Can you work these out from the model? Positions are in its coordinate system, mm. A direction names the side the tool comes from. Round coordinates to 2 decimals unless told otherwise and drop trailing zeros. Order: outer loops, then holes, each group sorted by start corner. A loop starts at its lowest first (then second) coordinate and runs counter-clockwise, first axis right, second up. Notation, with made-up numbers: (-37.5, -25.5) -> (-20.5, -25.5) arc R24 cw to (-20.5, -4.5) -> close; hole circle Ø9 at (64, 29.25). An arc over 180 degrees is marked (long way). One line per item, written item: value.
```python
from build123d import *

# Parameters (mm, degrees)
ESTRUSIONE_ESTRUSIONE1_DEPTH = 7.5
ESTRUSIONE_ESTRUSIONE2_DEPTH = 4
TAGLIO_ESTRUSIONE1_DEPTH     = 198.380910943
TAGLIO_ESTRUSIONE2_DEPTH     = 198.380910943
RACCORDO1_R                  = 25
TAGLIO_ESTRUSIONE3_DEPTH     = 7.5
TAGLIO_ESTRUSIONE4_DEPTH     = 7.5
SCHIZZO6_R                   = 3
TAGLIO_ESTRUSIONE5_DEPTH     = 198.380910943


with BuildPart() as part:
    # Schizzo1 → Estrusione-Estrusione1 (new, symmetric)
    with BuildSketch(Plane.XY):
        with BuildLine():
            Line((14.5, 182.011383906), (14.5, -37.988616094))
            ThreePointArc((14.5, -37.988616094), (0, -52.488616094), (-14.5, -37.988616094))
            Line((-14.5, -37.988616094), (-14.5, 182.011383906))
            ThreePointArc((-14.5, 182.011383906), (0, 196.511383906), (14.5, 182.011383906))
        make_face()
    extrude(amount=ESTRUSIONE_ESTRUSIONE1_DEPTH, both=True)

    # Schizzo2 → Estrusione-Estrusione2 (add, symmetric)
    with BuildSketch(Plane.XY):
        with BuildLine():
            Line((13, -40.066616094), (13, -56.066616094))
            ThreePointArc((13, -56.066616094), (0, -69.066616094), (-13, -56.066616094))
            Line((-13, -56.066616094), (-13, -40.066616094))
            ThreePointArc((-13, -40.066616094), (0, -27.066616094), (13, -40.066616094))
        make_face()
    extrude(amount=ESTRUSIONE_ESTRUSIONE2_DEPTH, both=True)

    # Schizzo4 → Taglio-Estrusione1 (cut, through all)
    with BuildSketch(Plane.XY.offset(4)):
        with BuildLine():
            Line((5.29445937, -51.487456784), (14.5, -37.988616094))
            Line((14.5, -37.988616094), (21.494330869, -44.738036439))
            Line((21.494330869, -44.738036439), (5.386515672, -60.537124892))
            ThreePointArc((5.386515672, -60.537124892), (0.071202698, -63.066253954), (-5.29445937, -60.645775404))
            Line((-5.29445937, -60.645775404), (-28.596127717, -39.453615031))
            Line((-28.596127717, -39.453615031), (-14.5, -31.562211214))
            Line((-14.5, -31.562211214), (-3.845832517, -50.217721134))
            ThreePointArc((-3.845832517, -50.217721134), (0.963165144, -49.133196093), (5.29445937, -51.487456784))
        make_face()
    taglio_estrusione1 = extrude(amount=TAGLIO_ESTRUSIONE1_DEPTH, mode=Mode.SUBTRACT)

    # Specchia1: Taglio-Estrusione1 across plane
    add(taglio_estrusione1.mirror(Plane.XY), mode=Mode.SUBTRACT)

    # Schizzo5 → Taglio-Estrusione2 (cut, through all)
    with BuildSketch(Plane.XY.offset(4)):
        Polygon((-13, -44.411232383), (-13, -34.188720036), (-15.056335757, -30.588064032), (-15.056335757, -43.619366988), align=None)
        Polygon((13, -44.411232383), (13, -40.188189356), (17.407959402, -33.724436261), (17.407959402, -44.411232383), align=None)
    extrude(amount=-TAGLIO_ESTRUSIONE2_DEPTH, mode=Mode.SUBTRACT)

    # Raccordo1
    # the kernel refuses this fillet: 25 mm, written as the material it takes off along each edge
    with BuildSketch(Plane(origin=(-14.5, -31.562211214, -24.089497944), x_dir=(0.4959240379913526, -0.8683659070589721, 0), z_dir=(0, 0, 1))) as raccordo1_piece_1_section:
        with BuildLine():
            CenterArc((RACCORDO1_R * 0.26543196711, RACCORDO1_R), RACCORDO1_R, 240.269299078, 29.730700922)
            Line((-RACCORDO1_R * 0.230492070882, RACCORDO1_R * 0.131634092941), (0, 0))
            Line((0, 0), (RACCORDO1_R * 0.26543196711, 0))
        make_face()
    raccordo1_piece_1 = extrude(amount=48.178995889, mode=Mode.PRIVATE)
    raccordo1_piece_1 = split(raccordo1_piece_1, bisect_by=Plane(origin=(-13, -35.788331904, -14.044748972), z_dir=(1, 0, 0)), keep=Keep.TOP, mode=Mode.PRIVATE)
    raccordo1_piece_1 = split(raccordo1_piece_1, bisect_by=Plane(origin=(-12.28179921, -35.788331904, -4), z_dir=(0, 0, -1)), keep=Keep.TOP, mode=Mode.PRIVATE)
    add(raccordo1_piece_1, mode=Mode.SUBTRACT)
    with BuildSketch(Plane(origin=(-14.5, -31.562211214, -24.089497944), x_dir=(0.4959240379913526, -0.8683659070589721, 0), z_dir=(0, 0, 1))) as raccordo1_piece_2_section:
        with BuildLine():
            CenterArc((RACCORDO1_R * 0.26543196711, RACCORDO1_R), RACCORDO1_R, 240.269299078, 29.730700922)
            Line((-RACCORDO1_R * 0.230492070882, RACCORDO1_R * 0.131634092941), (0, 0))
            Line((0, 0), (RACCORDO1_R * 0.26543196711, 0))
        make_face()
    raccordo1_piece_2 = extrude(amount=48.178995889, mode=Mode.PRIVATE)
    raccordo1_piece_2 = split(raccordo1_piece_2, bisect_by=Plane(origin=(-13, -30.370530988, -14.044748972), z_dir=(-1, 0, 0)), keep=Keep.TOP, mode=Mode.PRIVATE)
    raccordo1_piece_2 = split(raccordo1_piece_2, bisect_by=Plane(origin=(-14.266276842, -30.370530988, -4), z_dir=(0, 0, -1)), keep=Keep.TOP, mode=Mode.PRIVATE)
    add(raccordo1_piece_2, mode=Mode.SUBTRACT)
    with BuildSketch(Plane(origin=(-14.5, -31.562211214, -24.089497944), x_dir=(0.4959240379913526, -0.8683659070589721, 0), z_dir=(0, 0, 1))) as raccordo1_piece_3_section:
        with BuildLine():
            CenterArc((RACCORDO1_R * 0.26543196711, RACCORDO1_R), RACCORDO1_R, 240.269299078, 29.730700922)
            Line((-RACCORDO1_R * 0.230492070882, RACCORDO1_R * 0.131634092941), (0, 0))
            Line((0, 0), (RACCORDO1_R * 0.26543196711, 0))
        make_face()
    raccordo1_piece_3 = extrude(amount=48.178995889, mode=Mode.PRIVATE)
    raccordo1_piece_3 = split(raccordo1_piece_3, bisect_by=Plane(origin=(-14.266276842, -30.370530988, 4), z_dir=(0, 0, -1)), keep=Keep.TOP, mode=Mode.PRIVATE)
    raccordo1_piece_3 = split(raccordo1_piece_3, bisect_by=Plane(origin=(-13, -30.370530988, 0), z_dir=(-1, 0, 0)), keep=Keep.TOP, mode=Mode.PRIVATE)
    raccordo1_piece_3 = split(raccordo1_piece_3, bisect_by=Plane(origin=(-14.266276842, -30.370530988, -4), z_dir=(0, 0, 1)), keep=Keep.TOP, mode=Mode.PRIVATE)
    add(raccordo1_piece_3, mode=Mode.SUBTRACT)
    with BuildSketch(Plane(origin=(-14.5, -31.562211214, -24.089497944), x_dir=(0.4959240379913526, -0.8683659070589721, 0), z_dir=(0, 0, 1))) as raccordo1_piece_4_section:
        with BuildLine():
            CenterArc((RACCORDO1_R * 0.26543196711, RACCORDO1_R), RACCORDO1_R, 240.269299078, 29.730700922)
            Line((-RACCORDO1_R * 0.230492070882, RACCORDO1_R * 0.131634092941), (0, 0))
            Line((0, 0), (RACCORDO1_R * 0.26543196711, 0))
        make_face()
    raccordo1_piece_4 = extrude(amount=48.178995889, mode=Mode.PRIVATE)
    raccordo1_piece_4 = split(raccordo1_piece_4, bisect_by=Plane(origin=(-12.28179921, -35.788331904, 4), z_dir=(0, 0, 1)), keep=Keep.TOP, mode=Mode.PRIVATE)
    raccordo1_piece_4 = split(raccordo1_piece_4, bisect_by=Plane(origin=(-13, -35.788331904, 14.044748972), z_dir=(1, 0, 0)), keep=Keep.TOP, mode=Mode.PRIVATE)
    add(raccordo1_piece_4, mode=Mode.SUBTRACT)
    with BuildSketch(Plane(origin=(-14.5, -31.562211214, -24.089497944), x_dir=(0.4959240379913526, -0.8683659070589721, 0), z_dir=(0, 0, 1))) as raccordo1_piece_5_section:
        with BuildLine():
            CenterArc((RACCORDO1_R * 0.26543196711, RACCORDO1_R), RACCORDO1_R, 240.269299078, 29.730700922)
            Line((-RACCORDO1_R * 0.230492070882, RACCORDO1_R * 0.131634092941), (0, 0))
            Line((0, 0), (RACCORDO1_R * 0.26543196711, 0))
        make_face()
    raccordo1_piece_5 = extrude(amount=48.178995889, mode=Mode.PRIVATE)
    raccordo1_piece_5 = split(raccordo1_piece_5, bisect_by=Plane(origin=(-14.266276842, -30.370530988, 4), z_dir=(0, 0, 1)), keep=Keep.TOP, mode=Mode.PRIVATE)
    raccordo1_piece_5 = split(raccordo1_piece_5, bisect_by=Plane(origin=(-13, -30.370530988, 14.044748972), z_dir=(-1, 0, 0)), keep=Keep.TOP, mode=Mode.PRIVATE)
    add(raccordo1_piece_5, mode=Mode.SUBTRACT)
    with BuildSketch(Plane(origin=(14.5, -37.988616094, 26.782481556), x_dir=(0, 1, 0), z_dir=(0, 0, -1))) as raccordo1_piece_6_section:
        with BuildLine():
            CenterArc((RACCORDO1_R * 0.308519704891, -RACCORDO1_R), RACCORDO1_R, 90, 34.292050498)
            Line((-RACCORDO1_R * 0.254891721625, -RACCORDO1_R * 0.173823527041), (0, 0))
            Line((0, 0), (RACCORDO1_R * 0.308519704891, 0))
        make_face()
    raccordo1_piece_6 = extrude(amount=53.564963111, mode=Mode.PRIVATE)
    raccordo1_piece_6 = split(raccordo1_piece_6, bisect_by=Plane(origin=(14.242102238, -36.251699178, 4), z_dir=(0, 0, 1)), keep=Keep.TOP, mode=Mode.PRIVATE)
    raccordo1_piece_6 = split(raccordo1_piece_6, bisect_by=Plane(origin=(13, -36.251699178, 15.391240778), z_dir=(1, 0, 0)), keep=Keep.TOP, mode=Mode.PRIVATE)
    add(raccordo1_piece_6, mode=Mode.SUBTRACT)
    with BuildSketch(Plane(origin=(14.5, -37.988616094, 26.782481556), x_dir=(0, 1, 0), z_dir=(0, 0, -1))) as raccordo1_piece_7_section:
        with BuildLine():
            CenterArc((RACCORDO1_R * 0.308519704891, -RACCORDO1_R), RACCORDO1_R, 90, 34.292050498)
            Line((-RACCORDO1_R * 0.254891721625, -RACCORDO1_R * 0.173823527041), (0, 0))
            Line((0, 0), (RACCORDO1_R * 0.308519704891, 0))
        make_face()
    raccordo1_piece_7 = extrude(amount=53.564963111, mode=Mode.PRIVATE)
    raccordo1_piece_7 = split(raccordo1_piece_7, bisect_by=Plane(origin=(11.895384145, -41.966992208, 4), z_dir=(0, 0, 1)), keep=Keep.TOP, mode=Mode.PRIVATE)
    raccordo1_piece_7 = split(raccordo1_piece_7, bisect_by=Plane(origin=(13, -41.966992208, 15.391240778), z_dir=(-1, 0, 0)), keep=Keep.TOP, mode=Mode.PRIVATE)
    add(raccordo1_piece_7, mode=Mode.SUBTRACT)
    with BuildSketch(Plane(origin=(14.5, -37.988616094, 26.782481556), x_dir=(0, 1, 0), z_dir=(0, 0, -1))) as raccordo1_piece_8_section:
        with BuildLine():
            CenterArc((RACCORDO1_R * 0.308519704891, -RACCORDO1_R), RACCORDO1_R, 90, 34.292050498)
            Line((-RACCORDO1_R * 0.254891721625, -RACCORDO1_R * 0.173823527041), (0, 0))
            Line((0, 0), (RACCORDO1_R * 0.308519704891, 0))
        make_face()
    raccordo1_piece_8 = extrude(amount=53.564963111, mode=Mode.PRIVATE)
    raccordo1_piece_8 = split(raccordo1_piece_8, bisect_by=Plane(origin=(14.242102238, -36.251699178, 4), z_dir=(0, 0, -1)), keep=Keep.TOP, mode=Mode.PRIVATE)
    raccordo1_piece_8 = split(raccordo1_piece_8, bisect_by=Plane(origin=(14.242102238, -36.251699178, -4), z_dir=(0, 0, 1)), keep=Keep.TOP, mode=Mode.PRIVATE)
    raccordo1_piece_8 = split(raccordo1_piece_8, bisect_by=Plane(origin=(13, -36.251699178, 0), z_dir=(1, 0, 0)), keep=Keep.TOP, mode=Mode.PRIVATE)
    add(raccordo1_piece_8, mode=Mode.SUBTRACT)
    with BuildSketch(Plane(origin=(14.5, -37.988616094, 26.782481556), x_dir=(0, 1, 0), z_dir=(0, 0, -1))) as raccordo1_piece_9_section:
        with BuildLine():
            CenterArc((RACCORDO1_R * 0.308519704891, -RACCORDO1_R), RACCORDO1_R, 90, 34.292050498)
            Line((-RACCORDO1_R * 0.254891721625, -RACCORDO1_R * 0.173823527041), (0, 0))
            Line((0, 0), (RACCORDO1_R * 0.308519704891, 0))
        make_face()
    raccordo1_piece_9 = extrude(amount=53.564963111, mode=Mode.PRIVATE)
    raccordo1_piece_9 = split(raccordo1_piece_9, bisect_by=Plane(origin=(14.242102238, -36.251699178, -4), z_dir=(0, 0, -1)), keep=Keep.TOP, mode=Mode.PRIVATE)
    raccordo1_piece_9 = split(raccordo1_piece_9, bisect_by=Plane(origin=(13, -36.251699178, -15.391240778), z_dir=(1, 0, 0)), keep=Keep.TOP, mode=Mode.PRIVATE)
    add(raccordo1_piece_9, mode=Mode.SUBTRACT)
    with BuildSketch(Plane(origin=(14.5, -37.988616094, 26.782481556), x_dir=(0, 1, 0), z_dir=(0, 0, -1))) as raccordo1_piece_10_section:
        with BuildLine():
            CenterArc((RACCORDO1_R * 0.308519704891, -RACCORDO1_R), RACCORDO1_R, 90, 34.292050498)
            Line((-RACCORDO1_R * 0.254891721625, -RACCORDO1_R * 0.173823527041), (0, 0))
            Line((0, 0), (RACCORDO1_R * 0.308519704891, 0))
        make_face()
    raccordo1_piece_10 = extrude(amount=53.564963111, mode=Mode.PRIVATE)
    raccordo1_piece_10 = split(raccordo1_piece_10, bisect_by=Plane(origin=(11.895384145, -41.966992208, -4), z_dir=(0, 0, -1)), keep=Keep.TOP, mode=Mode.PRIVATE)
    raccordo1_piece_10 = split(raccordo1_piece_10, bisect_by=Plane(origin=(13, -41.966992208, -15.391240778), z_dir=(-1, 0, 0)), keep=Keep.TOP, mode=Mode.PRIVATE)
    add(raccordo1_piece_10, mode=Mode.SUBTRACT)

    # Schizzo8 → Taglio-Estrusione3 (cut, symmetric)
    with BuildSketch(Plane.XY):
        with BuildLine():
            Line((9, 182.011383906), (9, -27.988616094))
            ThreePointArc((9, -27.988616094), (0, -36.988616094), (-9, -27.988616094))
            Line((-9, -27.988616094), (-9, 182.011383906))
            ThreePointArc((-9, 182.011383906), (0, 191.011383906), (9, 182.011383906))
        make_face()
    extrude(amount=TAGLIO_ESTRUSIONE3_DEPTH, both=True, mode=Mode.SUBTRACT)

    # Schizzo9 → Taglio-Estrusione4 (cut)
    with BuildSketch(Plane.XY.offset(7.5)):
        with BuildLine():
            Line((-9, 182.011383906), (-9, 202.011383906))
            ThreePointArc((-9, 202.011383906), (0, 211.011383906), (9, 202.011383906))
            Line((9, 202.011383906), (9, 182.011383906))
            ThreePointArc((9, 182.011383906), (0, 173.011383906), (-9, 182.011383906))
        make_face()
    extrude(amount=-TAGLIO_ESTRUSIONE4_DEPTH, mode=Mode.SUBTRACT)

    # Schizzo6 → Taglio-Estrusione5 (cut, through all)
    with BuildSketch(Plane.XY.offset(4)):
        with Locations((0, -56.066616094)):
            Circle(SCHIZZO6_R)
    extrude(amount=-TAGLIO_ESTRUSIONE5_DEPTH, mode=Mode.SUBTRACT)


solid = part.part
```
Q1. I want a section at A-A on x = 0. List the corners of the cut face in (y, z) for me.
Answers below:
outline: (-69.07, -4) -> (-59.07, -4) -> (-59.07, 4) -> (-69.07, 4) -> close; (-53.07, -4) -> (-49.07, -4) -> (-49.07, -7.5) -> (-36.99, -7.5) -> (-36.99, 7.5) -> (-49.07, 7.5) -> (-49.07, 4) -> (-53.07, 4) -> close; (191.01, -7.5) -> (196.51, -7.5) -> (196.51, 0) -> (191.01, 0) -> close
Q2. Will these pins go through, and if not, where does the flat tip stop? pin 1 Ø9.5 at (x, y) = (0, -56.07) entering from +Z; pin 2 Ø3 at (x, z) = (-4.5, 4) entering from +Y; pin 3 Ø9 at (y, z) = (-43.5, -1) entering from +X.
Answers below:
pin 1: z = 4
pin 2: y = -34.7
pin 3: x = 13
Q3. We'd pull the mould along Y, two halves only. Please class faces 5 (the face through (-0.391, -53.092, 0.056)), 6 (the face through (-7.58, -43.68, -5.73)), 7 (the face through (-0.2, 191.01, -3.7)), 8 (the face through (-0.319, 196.508, -1.562)): released by +Y, released by -Y, zero draft, split by the parting line, or undercut.
Answers below:
face 5: undercut
face 6: released by -Y
face 7: undercut
face 8: released by +Y
Q4. On a 3-axis mill with a long thin cutter (end or side, diameter ignored), from which of +Z, -Z, +X, -X, +Y, -Y can I reach the whole of each face in a straight line? I mean faces 1 (the face through (13, -47, 0)), 2 (the face through (7.69, -47.974, 5.726)), 3 (the face through (3, -55, -4)), 4 (the face through (7.69, -47.974, -5.726)). Say none if no direction works.
Answers below:
face 1: +Z, -Z, +X, -Y
face 2: +Z, +X, -Y
face 3: -Z, -Y
face 4: -Z, +X, -Y
Q5. I want a section at B-B on y = 55. List the corners of the cut face in (x, z) for me.
Answers below:
outline: (-14.5, -7.5) -> (-9, -7.5) -> (-9, 7.5) -> (-14.5, 7.5) -> close; (9, -7.5) -> (14.5, -7.5) -> (14.5, 7.5) -> (9, 7.5) -> close
Q6. Please list where these lines run through material, in increasing order: line 1 along Y through (x, z) = (0, -0.25); line 2 along Y through (x, z) = (-1.5, -2); line 3 along X through (y, z) = (-14, -0.75).
Answers below:
line 1: -69.07 to -59.07, -53.07 to -36.99, 191.01 to 196.51
line 2: -68.98 to -58.66, -53.47 to -36.86, 190.89 to 196.43
line 3: -14.5 to -9, 9 to 14.5
